Check sheet for the modelled part. Datum: model origin and axes. Units: mm. A direction names the side the tool comes from. Coordinates: 2 decimals unless noted, no trailing zeros. Write each loop counter-clockwise with the first axis right and the second up, starting at its lowest first coordinate (ties: lowest second). Pieces come first, ordered by that corner, then holes. Notation, with made-up numbers: (81, 33.5) -> (125, 33.5) arc R24 cw to (125, 54.5) -> close; hole circle Ø8 at (23.25, -30). An arc over 180 degrees is marked (long way). One line per item, written item: value. Start each with the question number.
1) Draft check along Y on faces 4 (the cylindrical face through (10.5, -0.1, 6)), 5 (the cylindrical face through (0.35, 8.56, 3.94)), 6 (the flat face through (90, 0, 2)). Enter one of: +Y half, -Y half, draft (parallel to the pull), parting line (faces both ways), or undercut.
2) Sectioned sample at C-C on x = 27. Enter the section's corners in (y, z), plus the area to 3 significant figures.
3) Sectioned sample at D-D on y = -12. Enter the section's corners in (x, z).
4) Scan lines: line 1 along Y through (x, z) = (35, 1.05); line 2 along Y through (x, z) = (27, 1.2); line 3 along Y through (x, z) = (51, 0.85). Record each from-to range of solid material in increasing order. Write a range as [from, to].
5) Gauge pin test, flat ends, axial feed: P1, Ø3, axis at x = 64.5, z = 3, coming from the -Y side; P2, Ø3, axis at x = 64.5, z = 2, coming from the +Y side; P3, Ø4, axis at y = -6, z = 2, coming from the -X side. Record the tip position at first contact, or that the pin passes through.
6) Sectioned sample at A-A on x = 72. Enter the section's corners in (y, z).
7) Sectioned sample at B-B on z = 6.5. Enter the section's corners in (x, y) (3 decimals).
8) Set-up check for faces 1 (the cylindrical face through (-10.5, 0.1, 6)), 2 (the flat face through (66, -14, 2)), 3 (the flat face through (65, -6.5, 2)): record each of +Z, -Z, +X, -X, +Y, -Y from which the full face is reachable in a straight line by a thin tool's end or side.
```python
from build123d import *

# Parameters (mm, degrees)
MAIN_WEB_PROFILE_W                      = 60
MAIN_WEB_PROFILE_H                      = 14
MAIN_WEB_DEPTH                          = 4
SHOULDER_HORN_FLANGE_PROFILE_R          = 16
SHOULDER_HORN_FLANGE_DEPTH              = 4
ELBOW_SERVO_MOUNT_PROFILE_W             = 48
ELBOW_SERVO_MOUNT_PROFILE_H             = 28
ELBOW_SERVO_MOUNT_DEPTH                 = 4
SG90_BODY_CLEARANCE_START               = -5
SG90_BODY_CLEARANCE_PROFILE_W           = 23.8
SG90_BODY_CLEARANCE_PROFILE_H           = 13
SG90_BODY_CLEARANCE_DEPTH               = 97.49863387
ELBOW_TAB_FASTENERS_START               = -50
ELBOW_TAB_FASTENERS_PROFILE_R           = 1.3
ELBOW_TAB_FASTENERS_DEPTH               = 142.49863387
SHOULDER_CENTER_SCREW_ACCESS_START      = -50
SHOULDER_CENTER_SCREW_ACCESS_PROFILE_R  = 4
SHOULDER_CENTER_SCREW_ACCESS_DEPTH      = 142.49863387
CABLE_TIE_HOLES_START                   = -50
CABLE_TIE_HOLES_PROFILE_R               = 1.6
CABLE_TIE_HOLES_DEPTH                   = 142.49863387
PASSIVE_LOWER_MOUNT_BOSS_PROFILE_R      = 5
PASSIVE_LOWER_MOUNT_BOSS_DEPTH          = 4
PASSIVE_UPPER_MOUNT_BOSS_PROFILE_R      = 5
PASSIVE_UPPER_MOUNT_BOSS_DEPTH          = 4
PASSIVE_CHEEK_STANDOFFS_START           = -50
PASSIVE_CHEEK_STANDOFFS_PROFILE_R       = 1.6
PASSIVE_CHEEK_STANDOFFS_DEPTH           = 142.49863387
SHOULDER_DOWEL_SUPPORT_HUB_START        = 4
SHOULDER_DOWEL_SUPPORT_HUB_PROFILE_R    = 7
SHOULDER_DOWEL_SUPPORT_HUB_PROFILE_R_2  = 4
SHOULDER_DOWEL_SUPPORT_HUB_DEPTH        = 4
RAISED_M3_WASHER_SEATS_HEIGHT8_START    = 4
RAISED_M3_WASHER_SEATS_PCD14_PROFILE_R  = 3.5
RAISED_M3_WASHER_SEATS_HEIGHT8_DEPTH    = 4
METAL_HORN_M3_CLEARANCE_PCD14_START     = -50
METAL_HORN_M3_CLEARANCE_PCD14_PROFILE_R = 1.6
METAL_HORN_M3_CLEARANCE_PCD14_DEPTH     = 142.760557976
RESTORE_SHOULDER_SLEEVE_BORE_START      = -50
RESTORE_SHOULDER_SLEEVE_BORE_PROFILE_R  = 4
RESTORE_SHOULDER_SLEEVE_BORE_DEPTH      = 142.760557976


with BuildPart() as part:
    # Main_web_profile → Main_web (new body)
    with BuildSketch(Plane.XY):
        with Locations((30, 0)):
            Rectangle(MAIN_WEB_PROFILE_W, MAIN_WEB_PROFILE_H)
    extrude(amount=MAIN_WEB_DEPTH)

    # Shoulder_horn_flange_profile → Shoulder_horn_flange (add)
    with BuildSketch(Plane.XY):
        Circle(SHOULDER_HORN_FLANGE_PROFILE_R)
    extrude(amount=SHOULDER_HORN_FLANGE_DEPTH)

    # Elbow_servo_mount_profile → Elbow_servo_mount (add)
    with BuildSketch(Plane.XY):
        with Locations((66, 0)):
            Rectangle(ELBOW_SERVO_MOUNT_PROFILE_W, ELBOW_SERVO_MOUNT_PROFILE_H)
    extrude(amount=ELBOW_SERVO_MOUNT_DEPTH)

    # SG90_body_clearance_profile → SG90_body_clearance (cut, through all)
    with BuildSketch(Plane.XY.offset(SG90_BODY_CLEARANCE_START)):
        with Locations((65.5, 0)):
            Rectangle(SG90_BODY_CLEARANCE_PROFILE_W, SG90_BODY_CLEARANCE_PROFILE_H)
    extrude(amount=SG90_BODY_CLEARANCE_DEPTH, mode=Mode.SUBTRACT)

    # Elbow_tab_fasteners_profile → Elbow_tab_fasteners (cut, through all)
    with BuildSketch(Plane.XY.offset(ELBOW_TAB_FASTENERS_START)):
        with Locations(Location((51, 0, 0), (0, 0, 180))):
            Circle(ELBOW_TAB_FASTENERS_PROFILE_R)
        with Locations(Location((80, 0, 0), (0, 0, 180))):
            Circle(ELBOW_TAB_FASTENERS_PROFILE_R)
    extrude(amount=ELBOW_TAB_FASTENERS_DEPTH, mode=Mode.SUBTRACT)

    # Shoulder_center_screw_access_profile → Shoulder_center_screw_access (cut, through all)
    with BuildSketch(Plane.XY.offset(SHOULDER_CENTER_SCREW_ACCESS_START)):
        with Locations(Location((0, 0, 0), (0, 0, 180))):
            Circle(SHOULDER_CENTER_SCREW_ACCESS_PROFILE_R)
    extrude(amount=SHOULDER_CENTER_SCREW_ACCESS_DEPTH, mode=Mode.SUBTRACT)

    # Cable_tie_holes_profile → Cable_tie_holes (cut, through all)
    with BuildSketch(Plane.XY.offset(CABLE_TIE_HOLES_START)):
        with Locations(Location((27, -3, 0), (0, 0, 180))):
            Circle(CABLE_TIE_HOLES_PROFILE_R)
        with Locations(Location((27, 3, 0), (0, 0, 180))):
            Circle(CABLE_TIE_HOLES_PROFILE_R)
    extrude(amount=CABLE_TIE_HOLES_DEPTH, mode=Mode.SUBTRACT)

    # Passive_lower_mount_boss_profile → Passive_lower_mount_boss (add)
    with BuildSketch(Plane.XY):
        with Locations((35, -9)):
            Circle(PASSIVE_LOWER_MOUNT_BOSS_PROFILE_R)
    extrude(amount=PASSIVE_LOWER_MOUNT_BOSS_DEPTH)

    # Passive_upper_mount_boss_profile → Passive_upper_mount_boss (add)
    with BuildSketch(Plane.XY):
        with Locations((35, 9)):
            Circle(PASSIVE_UPPER_MOUNT_BOSS_PROFILE_R)
    extrude(amount=PASSIVE_UPPER_MOUNT_BOSS_DEPTH)

    # Passive_cheek_standoffs_profile → Passive_cheek_standoffs (cut, through all)
    with BuildSketch(Plane.XY.offset(PASSIVE_CHEEK_STANDOFFS_START)):
        with Locations(Location((35, -9, 0), (0, 0, 180))):
            Circle(PASSIVE_CHEEK_STANDOFFS_PROFILE_R)
        with Locations(Location((35, 9, 0), (0, 0, 180))):
            Circle(PASSIVE_CHEEK_STANDOFFS_PROFILE_R)
    extrude(amount=PASSIVE_CHEEK_STANDOFFS_DEPTH, mode=Mode.SUBTRACT)

    # Shoulder_dowel_support_hub_profile → Shoulder_dowel_support_hub (add)
    with BuildSketch(Plane.XY.offset(SHOULDER_DOWEL_SUPPORT_HUB_START)):
        Circle(SHOULDER_DOWEL_SUPPORT_HUB_PROFILE_R)
        with Locations(Location((0, 0, 0), (0, 0, 180))):
            Circle(SHOULDER_DOWEL_SUPPORT_HUB_PROFILE_R_2, mode=Mode.SUBTRACT)
    extrude(amount=SHOULDER_DOWEL_SUPPORT_HUB_DEPTH)

    # Raised_M3_washer_seats_PCD14_profile → Raised_M3_washer_seats_height8 (add)
    with BuildSketch(Plane.XY.offset(RAISED_M3_WASHER_SEATS_HEIGHT8_START)):
        with Locations((7, 0)):
            Circle(RAISED_M3_WASHER_SEATS_PCD14_PROFILE_R)
        with Locations((-7, 0)):
            Circle(RAISED_M3_WASHER_SEATS_PCD14_PROFILE_R)
        with Locations((0, 7)):
            Circle(RAISED_M3_WASHER_SEATS_PCD14_PROFILE_R)
        with Locations((0, -7)):
            Circle(RAISED_M3_WASHER_SEATS_PCD14_PROFILE_R)
    extrude(amount=RAISED_M3_WASHER_SEATS_HEIGHT8_DEPTH)

    # Metal_horn_M3_clearance_PCD14_profile → Metal_horn_M3_clearance_PCD14 (cut, through all)
    with BuildSketch(Plane.XY.offset(METAL_HORN_M3_CLEARANCE_PCD14_START)):
        with Locations(Location((7, 0, 0), (0, 0, 180))):
            Circle(METAL_HORN_M3_CLEARANCE_PCD14_PROFILE_R)
        with Locations(Location((-7, 0, 0), (0, 0, 180))):
            Circle(METAL_HORN_M3_CLEARANCE_PCD14_PROFILE_R)
        with Locations(Location((0, 7, 0), (0, 0, 180))):
            Circle(METAL_HORN_M3_CLEARANCE_PCD14_PROFILE_R)
        with Locations(Location((0, -7, 0), (0, 0, 180))):
            Circle(METAL_HORN_M3_CLEARANCE_PCD14_PROFILE_R)
    extrude(amount=METAL_HORN_M3_CLEARANCE_PCD14_DEPTH, mode=Mode.SUBTRACT)

    # Restore_shoulder_sleeve_bore_profile → Restore_shoulder_sleeve_bore (cut, through all)
    with BuildSketch(Plane.XY.offset(RESTORE_SHOULDER_SLEEVE_BORE_START)):
        with Locations(Location((0, 0, 0), (0, 0, 180))):
            Circle(RESTORE_SHOULDER_SLEEVE_BORE_PROFILE_R)
    extrude(amount=RESTORE_SHOULDER_SLEEVE_BORE_DEPTH, mode=Mode.SUBTRACT)


solid = part.part
```
Answers:
1. face 4: parting line
1. face 5: undercut
1. face 6: draft
2. outline: (-7, 0) -> (-4.6, 0) -> (-4.6, 4) -> (-7, 4) -> close; (-1.4, 0) -> (1.4, 0) -> (1.4, 4) -> (-1.4, 4) -> close; (4.6, 0) -> (7, 0) -> (7, 4) -> (4.6, 4) -> close
2. area: 30.4 mm2
3. outline: (-10.58, 0) -> (10.58, 0) -> (10.58, 4) -> (-10.58, 4) -> close; (31, 0) -> (39, 0) -> (39, 4) -> (31, 4) -> close; (42, 0) -> (90, 0) -> (90, 4) -> (42, 4) -> close
4. line 1: y = [-14, -10.6], [-7.4, 7.4], [10.6, 14]
4. line 2: y = [-7, -4.6], [-1.4, 1.4], [4.6, 7]
4. line 3: y = [-14, -1.3], [1.3, 14]
5. P1: stops at y = -14
5. P2: stops at y = 14
5. P3: stops at x = -15.49
6. outline: (-14, 0) -> (-6.5, 0) -> (-6.5, 4) -> (-14, 4) -> close; (6.5, 0) -> (14, 0) -> (14, 4) -> (6.5, 4) -> close
7. outline: (-6.125, -3.389) arc R7 ccw to (-3.389, -6.125) arc R3.5 ccw (long way) to (3.389, -6.125) arc R7 ccw to (6.125, -3.389) arc R3.5 ccw (long way) to (6.125, 3.389) arc R7 ccw to (3.389, 6.125) arc R3.5 ccw (long way) to (-3.389, 6.125) arc R7 ccw to (-6.125, 3.389) arc R3.5 ccw (long way) to start; hole circle Ø3.2 at (-7, 0); hole circle Ø8 at (0, 0); hole circle Ø3.2 at (0, -7); hole circle Ø3.2 at (0, 7); hole circle Ø3.2 at (7, 0)
8. face 1: +Z
8. face 2: +Z, -Z, +X, -Y
8. face 3: +Z, -Z
